```python
from build123d import *

# Parameters (mm, degrees)
SKETCH_1_R               = 31.5
SKETCH_1_R_2             = 30.5
EXTRUDE_1_DEPTH          = 60
SKETCH_2_W               = 31.5
SKETCH_2_H               = 1
EXTRUDE_1_2_DEPTH        = 10
PATTERN_CIRCULAR_1_COUNT = 8
SKETCH_3_R               = 12
EXTRUDE_2_DEPTH          = 3
SKETCH_4_R               = 1.6
SKETCH_4_R_2             = 5.1
CUT_EXTRUDE_1_DEPTH      = 5
PATTERN_CIRCULAR_3_COUNT = 2


with BuildPart() as part:
    # 草图1 → Extrude 1 (new body)
    with BuildSketch(Plane.XY):
        Circle(SKETCH_1_R)
        Circle(SKETCH_1_R_2, mode=Mode.SUBTRACT)
    extrude(amount=EXTRUDE_1_DEPTH)

    # 草图2 → Extrude 1 2 (add)
    with BuildSketch(Plane.XY):
        with Locations((15.75, -0.5)):
            Rectangle(SKETCH_2_W, SKETCH_2_H)
    extrude_1_2 = extrude(amount=EXTRUDE_1_2_DEPTH)

    # 阵列(圆周)1: Extrude 1 2 ×8 about axis
    pattern_circular_1_axis = Axis((0, 0, 0), (0, 0, 1))
    for i in range(1, PATTERN_CIRCULAR_1_COUNT):
        add(extrude_1_2.rotate(pattern_circular_1_axis, i * 360 / PATTERN_CIRCULAR_1_COUNT))

    # 草图3 → 凸台-拉伸2 (add)
    with BuildSketch(Plane.XY.offset(10)):
        Circle(SKETCH_3_R)
    extrude(amount=-EXTRUDE_2_DEPTH)

    # 草图4 → 切除-拉伸1 (cut)
    with BuildSketch(Plane(origin=(0, 0, 7), x_dir=(-1, 0, 0), z_dir=(0, 0, -1))):
        with Locations((-7.22609389, -3.432720072)):
            Circle(SKETCH_4_R)
        with Locations((4.076355085, -8.580986494)):
            Circle(SKETCH_4_R)
        with Locations(Location((0, 0, 0), (0, 0, 180))):
            Circle(SKETCH_4_R_2)
    cut_extrude_1 = extrude(amount=-CUT_EXTRUDE_1_DEPTH, mode=Mode.SUBTRACT)

    # 阵列(圆周)3: 切除-拉伸1 ×2 about axis
    pattern_circular_3_axis = Axis((0, 0, 0), (0, 0, 1))
    for i in range(1, PATTERN_CIRCULAR_3_COUNT):
        add(cut_extrude_1.rotate(pattern_circular_3_axis, i * 360 / PATTERN_CIRCULAR_3_COUNT), mode=Mode.SUBTRACT)


solid = part.part
```
Model file for the job. Use its own axes, mm. A direction names the side the tool comes from. Coordinates: 2 decimals unless noted, no trailing zeros. Order: outer loops, then holes, each group sorted by start corner. A loop starts at its lowest first (then second) coordinate and runs counter-clockwise, first axis right, second up. Notation, with made-up numbers: (8, -24) -> (19, -24) arc R13 cw to (19, -19) -> close; hole circle Ø8 at (12.5, 22). An arc over 180 degrees is marked (long way). Answer as a JSON object with one key per item and string values. Group by question number.
1) Cut at B-B, the plane y = -18.5. Write the cut outline in (x, z).
2) Which spindle directions (+Z, -Z, +X, -X, +Y, -Y) get a long thin tool onto all of the face, cutting with end or side? Do faces 3 (the face through (5.104, 10.86, 8.521)), 4 (the face through (9, -5, 7)). Say none if no direction does.
3) Flat gauge pins, fed straight in: pin 1 (6 mm diameter, centred on x = 18, y = 20.5, fed in from +Z); pin 2 (2 mm diameter, centred on x = 15, z = 52.5, fed in from +Y); pin 3 (3 mm diameter, centred on x = -19, z = 4, fed in from -Y); pin 4 (6 mm diameter, centred on x = -6, y = 6, fed in from -Z). Where does each tip first touch, or does it go through?
4) Drill centre lines: L1, parallel to X at y = 27.5, z = 6; L2, parallel to Y at x = 9.5, z = 9.5; L3, parallel to Y at x = 0, z = 29.5. Where is each one in solid material? Low to high.
5) Cut at C-C, the plane z = 36. Write the cut outline in (x, y).
6) Cut at A-A, the plane y = -6. Write the cut outline in (x, z), then the cut area to 3 significant figures.
7) Pull direction Y, two halves, no side cores. Call faces 1 (the face through (11, 11, 5)), 2 (the face through (16, -1, 5)): +Y half, -Y half, draft (parallel to the pull), parting line (faces both ways), or undercut.
Check values:
{
 "1": {"outline": "(-25.5, 0) -> (-24.25, 0) -> (-24.25, 60) -> (-25.5, 60) -> close; (-19.91, 0) -> (-18.5, 0) -> (-18.5, 10) -> (-19.91, 10) -> close; (-1, 0) -> (0, 0) -> (0, 10) -> (-1, 10) -> close; (17.09, 0) -> (18.5, 0) -> (18.5, 10) -> (17.09, 10) -> close; (24.25, 0) -> (25.5, 0) -> (25.5, 60) -> (24.25, 60) -> close"},
 "2": {"face 3": "+Z, -Z", "face 4": "-Z"},
 "3": {"pin 1": "stops at z = 10", "pin 2": "stops at y = 28.22", "pin 3": "stops at y = -26.19", "pin 4": "stops at z = 0"},
 "4": {"L1": "x = -15.36 to -13.19, 0 to 1, 13.19 to 15.36", "L2": "y = -30.03 to -28.98, -10.91 to -9.5, -7.33 to 7.33, 8.09 to 9.5, 28.98 to 30.03", "L3": "y = -31.5 to -30.5, 30.5 to 31.5"},
 "5": {"outline": "circle Ø63 at (0, 0); hole circle Ø61 at (0, 0)"},
 "6": {"outline": "(-30.92, 0) -> (-29.9, 0) -> (-29.9, 60) -> (-30.92, 60) -> close; (-10.39, 7) -> (-7.41, 7) -> (-7.41, 0) -> (-6, 0) -> (-6, 7) -> (-1, 7) -> (-1, 0) -> (0, 0) -> (0, 7) -> (4.59, 7) -> (4.59, 0) -> (6, 0) -> (6, 7) -> (10.39, 7) -> (10.39, 10) -> (-10.39, 10) -> close; (29.9, 0) -> (30.92, 0) -> (30.92, 60) -> (29.9, 60) -> close", "area": "211 mm²"},
 "7": {"face 1": "undercut", "face 2": "undercut"}
}
